Read the model definition and answer for the solid it produces. Units are mm, in the model's axes. A direction names the side the tool comes from. Round coordinates to 2 decimals unless told otherwise and drop trailing zeros. Write each loop counter-clockwise with the first axis right and the second up, starting at its lowest first coordinate (ties: lowest second). Pieces come first, ordered by that corner, then holes. Notation, with made-up numbers: (29, 16.5) - (88, 16.5) arc R32 ccw to (88, 45.5) - close; hole circle Ø9 at (85, 78). An arc over 180 degrees is marked (long way). One line per item, written item: value. Start each with the question number.
(1) Find the intervals of material crossed by L1, parallel to Z at x = 53, y = 14.75; L2, parallel to Z at x = 71, y = 8.5, in increasing order.
(2) Flat-ended cylindrical pins translate along their axes: pin 1 Ø6 at (x, y) = (16.5, 11) entering from -Z; pin 2 Ø1.5 at (x, z) = (6, -7) entering from +Y; pin 3 Ø12 at (y, z) = (17.5, 1.5) entering from +X; pin 4 Ø12 at (x, y) = (2, 4) entering from +Z. Find the tip coordinate at first contact, or state that the pin passes through.
(3) A cutting plane is placed at C-C, the plane z = 5.75. Determine the outline of the cut face in (x, y).
(4) A cutting plane is placed at A-A, the plane y = 15.5. Determine the outline of the cut face in (x, z).
(5) For faces 1 (the face through (30, 10, 0)), 2 (the face through (30, 10, -5)), 3 (the face through (-25, 10, -12)), determine the directions among +Z, -Z, +X, -X, +Y, -Y from which every point of the face is accessible in a straight line to the end or side of a thin tool.
(6) A cutting plane is placed at B-B, the plane x = 5. Determine the outline of the cut face in (y, z), plus the area to 3 significant figures.
from build123d import *

# Parameters (mm, degrees)
SKETCH_1_W      = 60
SKETCH_1_H      = 5
EXTRUDE_1_DEPTH = 20


with BuildPart() as part:
    # 草图1 → 凸台-拉伸1 (new body)
    with BuildSketch(Plane(origin=(0, 0, 0), x_dir=(1, 0, 0), z_dir=(0, 1, 0))):
        Polygon((-25, 9.099255857), (-25, 14.099255857), (0, 5), (0, 0), align=None)
        with Locations((30, 2.5)):
            Rectangle(SKETCH_1_W, SKETCH_1_H)
        Polygon((60, 0), (85, -9.099255857), (85, -4.099255857), (60, 5), align=None)
    extrude(amount=EXTRUDE_1_DEPTH)


solid = part.part
Here are the results:
1. L1: -5 to 0
1. L2: -1 to 4
2. pin 1: z = -5
2. pin 2: through
2. pin 3: x = 85
2. pin 4: z = 0
3. outline: (75.8, 0) - (85, 0) - (85, 20) - (75.8, 20) - close
4. outline: (-25, -14.1) - (0, -5) - (60, -5) - (85, 4.1) - (85, 9.1) - (60, 0) - (0, 0) - (-25, -9.1) - close
5. face 1: +Z, -X, +Y, -Y
5. face 2: -Z, +X, +Y, -Y
5. face 3: +Z, -Z, -X, +Y, -Y
6. outline: (0, -5) - (20, -5) - (20, 0) - (0, 0) - close
6. area: 100 mm²
